```python
from build123d import *

# Parameters (mm, degrees)
SKETCH1_W           = 133.500000388
SKETCH1_H           = 84
BOSS_EXTRUDE1_DEPTH = 3
SKETCH2_W           = 20
SKETCH2_H           = 3
CUT_EXTRUDE1_DEPTH  = 104.014399147
SKETCH3_W           = 3
SKETCH3_H           = 30
BOSS_EXTRUDE2_DEPTH = 3
SKETCH4_W           = 3
SKETCH4_H           = 3.4
CUT_EXTRUDE2_DEPTH  = 106.612611798


with BuildPart() as part:
    # Sketch1 → Boss-Extrude1 (new body)
    with BuildSketch(Plane(origin=(0, 0, 0), x_dir=(1, 0, 0), z_dir=(0, 1, 0))):
        with Locations((22.092889694, -10.056770433)):
            Rectangle(SKETCH1_W, SKETCH1_H)
    extrude(amount=BOSS_EXTRUDE1_DEPTH)

    # Sketch2 → Cut-Extrude1 (cut, through all)
    with BuildSketch(Plane.XZ):
        with Locations((63.842889888, 46.556770433)):
            Rectangle(SKETCH2_W, SKETCH2_H)
        with Locations((-19.6571105, 46.556770433)):
            Rectangle(SKETCH2_W, SKETCH2_H)
        with Locations((-19.6571105, -26.443229567)):
            Rectangle(SKETCH2_W, SKETCH2_H)
        with Locations((63.842889888, -26.443229567)):
            Rectangle(SKETCH2_W, SKETCH2_H)
    extrude(amount=-CUT_EXTRUDE1_DEPTH, mode=Mode.SUBTRACT)

    # Sketch3 → Boss-Extrude2 (add, through all)
    with BuildSketch(Plane.XZ):
        with Locations((90.342889888, 10.056770433)):
            Rectangle(SKETCH3_W, SKETCH3_H)
        with Locations((-46.1571105, 10.056770433)):
            Rectangle(SKETCH3_W, SKETCH3_H)
    extrude(amount=-BOSS_EXTRUDE2_DEPTH)

    # Sketch4 → Cut-Extrude2 (cut, symmetric)
    with BuildSketch(Plane.XZ):
        Polygon((88.842889888, 8.356770433), (88.842889888, 5.056770433), (91.842889888, 5.056770433), (91.842889888, 15.056770433), (88.842889888, 15.056770433), (88.842889888, 11.756770433), align=None)
        with Locations((87.342889888, 10.056770433)):
            Rectangle(SKETCH4_W, SKETCH4_H)
        Polygon((85.842889888, 7.156770433), (85.842889888, 8.356770433), (85.842889888, 11.756770433), (85.842889888, 12.956770433), (82.842889888, 12.956770433), (82.842889888, 11.756770433), (82.842889888, 8.356770433), (82.842889888, 7.156770433), align=None)
        with Locations((81.342889888, 10.056770433)):
            Rectangle(SKETCH4_W, SKETCH4_H)
    cut_extrude2 = extrude(amount=CUT_EXTRUDE2_DEPTH, both=True, mode=Mode.SUBTRACT)

    # Mirror1: Cut-Extrude2 across plane
    add(cut_extrude2.mirror(Plane(origin=(22.092889694, 0, 0), x_dir=(0, 0, 1), z_dir=(1, 0, 0))), mode=Mode.SUBTRACT)


solid = part.part
```
Model file for the job. Use its own axes, mm. A direction names the side the tool comes from. Coordinates: 2 decimals unless noted, no trailing zeros. Loops run counter-clockwise (first coordinate to the right, second up) from the corner with the lowest first, then second, coordinate; pieces in that order, holes last. Notation, with made-up numbers: M 76,16.5 L 126,16.5 A27 cw 126,48.5 Z; hole C -17,47.25 d7. An arc over 180 degrees is marked long. Use CSV: the item, a comma, the result in double quotes. Start each with the question number.
1. Flat gauge pins, fed straight in: pin 1 (8 mm diameter, centred on x = -2.5, z = -17.5, fed in from -Y); pin 2 (0.9 mm diameter, centred on y = 2, z = 7, fed in from -X); pin 3 (0.6 mm diameter, centred on y = 2, z = 12.5, fed in from +X). Where does each tip first touch, or does it go through?
2. Band-saw the part on A-A, the plane x = -17.5. List the corners of the cut face in (y, z).
3. Two-plate mould, pull along Z, no slides. Class faces 1 (the flat face through (90, 1, -4.943)), 2 (the flat face through (-20, 1, -27.943)), 3 (the flat face through (-47.657, 1, 20)), 4 (the flat face through (-44.657, 1, 13)): pulls with the +Z half, pulls with the -Z half, needs draft (parallel to the pull), parting line crosses it, or undercut.
4. Tool access for faces 5 (the flat face through (-46, 1, 15.057)), 6 (the flat face through (53.843, 1, 47)), 7 (the flat face through (88.843, 1, 7)): list every direction of +Z, -Z, +X, -X, +Y, -Y with a clear straight run to the whole face (end or side of a thin tool).
5. Band-saw the part on B-B, the plane z = 40. List the corners of the cut face in (x, y).
6. Band-saw the part on C-C, the plane y = 0.6. Give the number of separate pieces and of enclosed holes in the cut face, then the cut area to 3 significant figures.
7. Probe probe 1 along Z at (x, y) = (62, 0.7); probe 2 along X at (y, z) = (0.9, 48); probe 3 along Z at (x, y) = (81.5, 1.9). List the from-to ranges inside material, lowest first. Write a range as [from, to].
Entries:
1,pin 1,"stops at y = 0"
1,pin 2,"stops at x = -44.66"
1,pin 3,"stops at x = 88.84"
2,outline,"M 0,-31.94 L 3,-31.94 L 3,-27.94 L 0,-27.94 Z; M 0,-24.94 L 3,-24.94 L 3,45.06 L 0,45.06 Z; M 0,48.06 L 3,48.06 L 3,52.06 L 0,52.06 Z"
3,face 1,"pulls with the -Z half"
3,face 2,"undercut"
3,face 3,"needs draft"
3,face 4,"undercut"
4,face 5,"-X, +Y, -Y"
4,face 6,"+Y, -Y"
4,face 7,"+X, +Y, -Y"
5,outline,"M -44.66,0 L 88.84,0 L 88.84,3 L -44.66,3 Z"
6,separate pieces,"1"
6,enclosed holes,"4"
6,area,"11,000 mm2"
7,probe 1,"z = [-31.94, -27.94], [-24.94, 45.06], [48.06, 52.06]"
7,probe 2,"x = [-44.66, -29.66], [-9.66, 53.84], [73.84, 88.84]"
7,probe 3,"z = [-31.94, 8.36], [11.76, 52.06]"
